from build123d import *

# Parameters (mm, degrees)
F0_R     = 4.5
F1_DEPTH = 5


with BuildPart() as f1:
    # F0 (on Top) → F1 (new body)
    with BuildSketch(Plane.XY):
        with Locations((0.1191368252, -0.0813986216)):
            Circle(F0_R)
        with BuildLine():
            ThreePointArc((2.8198227273, 1.224853903), (2.8907754227, 1.0666516755), (2.9524701585, 0.9046146756))
            ThreePointArc((2.9524701585, 0.9046146756), (3.7646340496, 0.6823639942), (4.1191368252, -0.0813986216))
            ThreePointArc((4.1191368252, -0.0813986216), (3.7646340496, -0.8451612374), (2.9524701585, -1.0674119188))
            ThreePointArc((2.9524701585, -1.0674119188), (2.8907754227, -1.2294489187), (2.8198227273, -1.3876511462))
            ThreePointArc((2.8198227273, -1.3876511462), (3.129098142, -1.7441154101), (3.2404571688, -2.2027189652))
            ThreePointArc((3.2404571688, -2.2027189652), (2.5445395433, -3.155364707), (1.4253893498, -2.7820845237))
            ThreePointArc((1.4253893498, -2.7820845237), (1.2671871223, -2.8530372191), (1.1051501224, -2.9147319549))
            ThreePointArc((1.1051501224, -2.9147319549), (1.1156340147, -2.9977723613), (1.1191368252, -3.0813986216))
            ThreePointArc((1.1191368252, -3.0813986216), (0.0355105649, -4.0778958111), (-0.866876472, -2.9147319549))
            ThreePointArc((-0.866876472, -2.9147319549), (-1.0289134719, -2.8530372191), (-1.1871156994, -2.7820845237))
            ThreePointArc((-1.1871156994, -2.7820845237), (-2.7092902995, -2.9098257463), (-2.5815490769, -1.3876511462))
            ThreePointArc((-2.5815490769, -1.3876511462), (-2.6525017723, -1.2294489187), (-2.7141965081, -1.0674119188))
            ThreePointArc((-2.7141965081, -1.0674119188), (-3.8808631748, -0.0813986216), (-2.7141965081, 0.9046146756))
            ThreePointArc((-2.7141965081, 0.9046146756), (-2.6525017723, 1.0666516755), (-2.5815490769, 1.224853903))
            ThreePointArc((-2.5815490769, 1.224853903), (-2.7092902995, 2.7470285031), (-1.1871156994, 2.6192872805))
            ThreePointArc((-1.1871156994, 2.6192872805), (-1.0289134719, 2.6902399759), (-0.866876472, 2.7519347117))
            ThreePointArc((-0.866876472, 2.7519347117), (0.0355105649, 3.9150985679), (1.1191368252, 2.9186013784))
            ThreePointArc((1.1191368252, 2.9186013784), (1.1156340147, 2.8349751181), (1.1051501224, 2.7519347117))
            ThreePointArc((1.1051501224, 2.7519347117), (1.2671871223, 2.6902399759), (1.4253893498, 2.6192872805))
            ThreePointArc((1.4253893498, 2.6192872805), (2.5445395433, 2.9925674638), (3.2404571688, 2.039921722))
            ThreePointArc((3.2404571688, 2.039921722), (3.129098142, 1.5813181669), (2.8198227273, 1.224853903))
        make_face(mode=Mode.SUBTRACT)
        with BuildLine():
            ThreePointArc((2.9524701585, -1.0674119188), (3.0771767168, -0.5813986216), (3.1191368252, -0.0813986216))
            ThreePointArc((3.1191368252, -0.0813986216), (3.0771767168, 0.4186013784), (2.9524701585, 0.9046146756))
            ThreePointArc((2.9524701585, 0.9046146756), (2.1191368252, -0.0813986216), (2.9524701585, -1.0674119188))
        make_face()
        with BuildLine():
            ThreePointArc((2.9524701585, 0.9046146756), (3.0771767168, 0.4186013784), (3.1191368252, -0.0813986216))
            ThreePointArc((3.1191368252, -0.0813986216), (3.0771767168, -0.5813986216), (2.9524701585, -1.0674119188))
            ThreePointArc((2.9524701585, -1.0674119188), (3.7646340496, -0.8451612374), (4.1191368252, -0.0813986216))
            ThreePointArc((4.1191368252, -0.0813986216), (3.7646340496, 0.6823639942), (2.9524701585, 0.9046146756))
        make_face()
        with BuildLine():
            ThreePointArc((1.4253893498, 2.6192872805), (1.5333503876, 1.3328149408), (2.8198227273, 1.224853903))
            ThreePointArc((2.8198227273, 1.224853903), (2.2404571688, 2.039921722), (1.4253893498, 2.6192872805))
        make_face()
        with BuildLine():
            ThreePointArc((1.4253893498, 2.6192872805), (2.2404571688, 2.039921722), (2.8198227273, 1.224853903))
            ThreePointArc((2.8198227273, 1.224853903), (3.129098142, 1.5813181669), (3.2404571688, 2.039921722))
            ThreePointArc((3.2404571688, 2.039921722), (2.5445395433, 2.9925674638), (1.4253893498, 2.6192872805))
        make_face()
        with BuildLine():
            ThreePointArc((3.2404571688, -2.2027189652), (3.129098142, -1.7441154101), (2.8198227273, -1.3876511462))
            ThreePointArc((2.8198227273, -1.3876511462), (2.2404571688, -2.2027189652), (1.4253893498, -2.7820845237))
            ThreePointArc((1.4253893498, -2.7820845237), (2.5445395433, -3.155364707), (3.2404571688, -2.2027189652))
        make_face()
        with BuildLine():
            ThreePointArc((1.4253893498, -2.7820845237), (2.2404571688, -2.2027189652), (2.8198227273, -1.3876511462))
            ThreePointArc((2.8198227273, -1.3876511462), (1.5333503876, -1.495612184), (1.4253893498, -2.7820845237))
        make_face()
        with BuildLine():
            ThreePointArc((-0.866876472, 2.7519347117), (0.1191368252, 1.9186013784), (1.1051501224, 2.7519347117))
            ThreePointArc((1.1051501224, 2.7519347117), (0.1191368252, 2.9186013784), (-0.866876472, 2.7519347117))
        make_face()
        with BuildLine():
            ThreePointArc((-0.866876472, 2.7519347117), (0.1191368252, 2.9186013784), (1.1051501224, 2.7519347117))
            ThreePointArc((1.1051501224, 2.7519347117), (1.1156340147, 2.8349751181), (1.1191368252, 2.9186013784))
            ThreePointArc((1.1191368252, 2.9186013784), (0.0355105649, 3.9150985679), (-0.866876472, 2.7519347117))
        make_face()
        with BuildLine():
            ThreePointArc((1.1191368252, -3.0813986216), (1.1156340147, -2.9977723613), (1.1051501224, -2.9147319549))
            ThreePointArc((1.1051501224, -2.9147319549), (0.1191368252, -3.0813986216), (-0.866876472, -2.9147319549))
            ThreePointArc((-0.866876472, -2.9147319549), (0.0355105649, -4.0778958111), (1.1191368252, -3.0813986216))
        make_face()
        with BuildLine():
            ThreePointArc((-0.866876472, -2.9147319549), (0.1191368252, -3.0813986216), (1.1051501224, -2.9147319549))
            ThreePointArc((1.1051501224, -2.9147319549), (0.1191368252, -2.0813986216), (-0.866876472, -2.9147319549))
        make_face()
        with BuildLine():
            ThreePointArc((-1.0021835184, 2.039921722), (-1.0495377765, 2.3440040965), (-1.1871156994, 2.6192872805))
            ThreePointArc((-1.1871156994, 2.6192872805), (-2.0021835184, 2.039921722), (-2.5815490769, 1.224853903))
            ThreePointArc((-2.5815490769, 1.224853903), (-1.5435799633, 1.1512807487), (-1.0021835184, 2.039921722))
        make_face()
        with BuildLine():
            ThreePointArc((-2.5815490769, 1.224853903), (-2.0021835184, 2.039921722), (-1.1871156994, 2.6192872805))
            ThreePointArc((-1.1871156994, 2.6192872805), (-2.7092902995, 2.7470285031), (-2.5815490769, 1.224853903))
        make_face()
        with BuildLine():
            ThreePointArc((-2.5815490769, -1.3876511462), (-2.7092902995, -2.9098257463), (-1.1871156994, -2.7820845237))
            ThreePointArc((-1.1871156994, -2.7820845237), (-2.0021835184, -2.2027189652), (-2.5815490769, -1.3876511462))
        make_face()
        with BuildLine():
            ThreePointArc((-2.5815490769, -1.3876511462), (-2.0021835184, -2.2027189652), (-1.1871156994, -2.7820845237))
            ThreePointArc((-1.1871156994, -2.7820845237), (-1.0495377765, -2.5068013397), (-1.0021835184, -2.2027189652))
            ThreePointArc((-1.0021835184, -2.2027189652), (-1.5435799633, -1.3140779919), (-2.5815490769, -1.3876511462))
        make_face()
        with BuildLine():
            ThreePointArc((-1.8808631748, -0.0813986216), (-2.117100559, 0.5640986028), (-2.7141965081, 0.9046146756))
            ThreePointArc((-2.7141965081, 0.9046146756), (-2.8808631748, -0.0813986216), (-2.7141965081, -1.0674119188))
            ThreePointArc((-2.7141965081, -1.0674119188), (-2.117100559, -0.726895846), (-1.8808631748, -0.0813986216))
        make_face()
        with BuildLine():
            ThreePointArc((-2.7141965081, -1.0674119188), (-2.8808631748, -0.0813986216), (-2.7141965081, 0.9046146756))
            ThreePointArc((-2.7141965081, 0.9046146756), (-3.8808631748, -0.0813986216), (-2.7141965081, -1.0674119188))
        make_face()
    extrude(amount=F1_DEPTH)


solid = f1.part
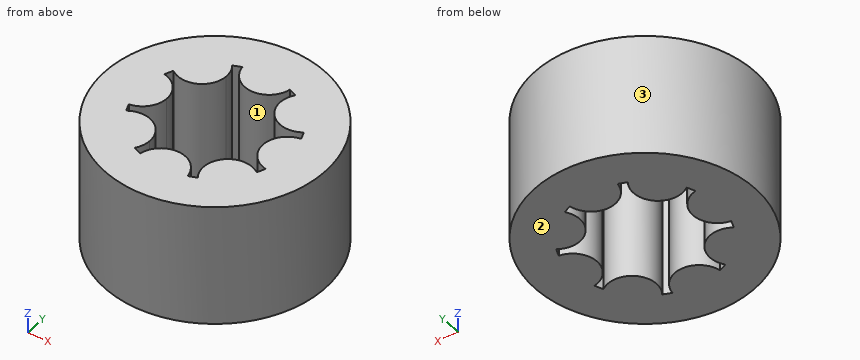
Geometry: final body of the model. Coordinates: model frame, mm. Face numbers are marked on the shaded views. Coordinates: 2 decimals unless noted, no trailing zeros. Order: outer loops, then holes, each group sorted by start corner. A loop starts at its lowest first (then second) coordinate and runs counter-clockwise, first axis right, second up.
(1) Draft query along X for the marked faces 1, 2 and 3. Return one class per face: pulls with the +X half, pulls with the -X half, needs draft (parallel to the pull), parting line crosses it, or undercut.
(2) Section query B-B (x = 2.5). Return the cut outline in (y, z), plus the area to 3 significant figures.
(3) Section query C-C (x = -1.5). Return the cut outline in (y, z), plus the area to 3 significant figures.
(4) Section query A-A (z = 1.6). Return the cut outline in (x, y), plus the area to 3 significant figures.
(5) Material intervals for probe 1 along X at (y, z) = (2.25, 2.25); probe 2 along X at (y, z) = (0, 2.9); probe 3 along Y at (x, z) = (-2, 3.4), sorted ascending.
(6) First-contact query: pin 1 (1 mm diameter, centred on x = -1.5, y = -1.5, fed in from -Z); pin 2 (3 mm diameter, centred on x = 2, z = 4, fed in from +Y). Flat tips, straight axial feed; report the tip coordinate or a pass-through.
(7) Section query D-D (y = 0.5). Return the cut outline in (x, z).
Solution:
1. face 1: undercut
1. face 2: needs draft
1. face 3: parting line crosses it
2. outline: (-3.9, 0) - (-1.24, 0) - (-1.24, 5) - (-3.9, 5) - close; (-0.87, 0) - (0.7, 0) - (0.7, 5) - (-0.87, 5) - close; (1.07, 0) - (3.74, 0) - (3.74, 5) - (1.07, 5) - close
2. area: 34.5 mm2
3. outline: (-4.28, 0) - (-1.34, 0) - (-1.34, 5) - (-4.28, 5) - close; (1.18, 0) - (4.12, 0) - (4.12, 5) - (1.18, 5) - close
3. area: 29.4 mm2
4. outline: circle Ø9 at (0.12, -0.08); hole (-2.71, -1.07) arc R3 ccw to (-2.58, -1.39) arc R1 cw to (-1.19, -2.78) arc R3 ccw to (-0.87, -2.91) arc R1 cw to (1.11, -2.91) arc R3 ccw to (1.43, -2.78) arc R1 cw to (2.82, -1.39) arc R3 ccw to (2.95, -1.07) arc R1 cw to (2.95, 0.9) arc R3 ccw to (2.82, 1.22) arc R1 cw to (1.43, 2.62) arc R3 ccw to (1.11, 2.75) arc R1 cw to (-0.87, 2.75) arc R3 ccw to (-1.19, 2.62) arc R1 cw to (-2.58, 1.22) arc R3 ccw to (-2.71, 0.9) arc R1 cw to start
4. area: 47.0 mm2
5. probe 1: x = -3.73 to -1.02, -0.62 to 0.86, 1.26 to 3.97
5. probe 2: x = -4.38 to -1.88, 2.12 to 4.62
5. probe 3: y = -4.05 to -1.2, -0.55 to 0.39, 1.04 to 3.89
6. pin 1: stops at z = 0
6. pin 2: stops at y = 4.4
7. outline: (-4.34, 0) - (-2.07, 0) - (-2.07, 5) - (-4.34, 5) - close; (2.31, 0) - (4.58, 0) - (4.58, 5) - (2.31, 5) - close
